from build123d import *

# Parameters (mm, degrees)
ESQUISSE1_R        = 1.5
ESQUISSE1_W        = 7.5
ESQUISSE1_H        = 5
BOSS_EXTRU_1_DEPTH = 5


with BuildPart() as part:
    # Esquisse1 → Boss.-Extru.1 (new body)
    with BuildSketch(Plane.XY):
        with BuildLine():
            Line((40, -6), (0, -6))
            ThreePointArc((0, -6), (-6, 0), (0, 6))
            Line((0, 6), (40, 6))
            ThreePointArc((40, 6), (46, 0), (40, -6))
        make_face()
        with Locations((40, 0)):
            Circle(ESQUISSE1_R, mode=Mode.SUBTRACT)
        Circle(ESQUISSE1_R, mode=Mode.SUBTRACT)
        with Locations((26.25, 0)):
            Rectangle(ESQUISSE1_W, ESQUISSE1_H, mode=Mode.SUBTRACT)
        with Locations((13.75, 0)):
            Rectangle(ESQUISSE1_W, ESQUISSE1_H, mode=Mode.SUBTRACT)
    extrude(amount=BOSS_EXTRU_1_DEPTH)


solid = part.part
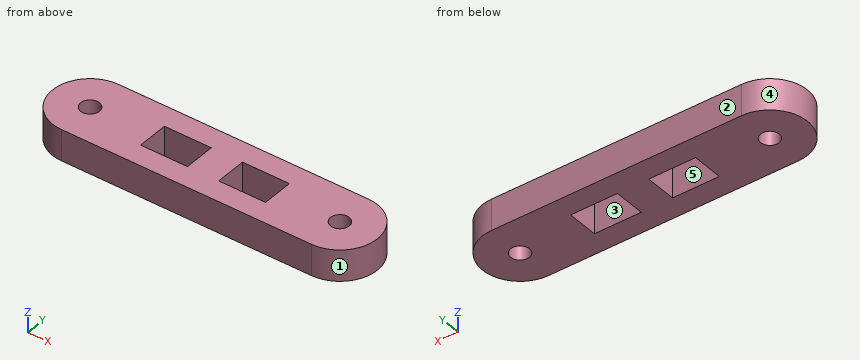
For this review, take the finished solid that the model builds, in its own axes (mm). Face numbers are marked on the shaded views. A direction names the side the tool comes from. Give positions to 0.01 mm unless a question says otherwise; leave off trailing zeros. Loops run counter-clockwise (first coordinate to the right, second up) from the corner with the lowest first, then second, coordinate; pieces in that order, holes last. Notation, with made-up numbers: M -25,45.25 L 10,45.25 A16 ccw 10,59.25 Z; hole C 76,49.5 d1. An arc over 180 degrees is marked long. Answer as a JSON object with one key per item and string values. Group by question number.
Q1. Add section A-A on y = 0. Give the boundary of the cut face in (x, z), and give its area (3 significant figures).
Q2. Tool access review of the marked faces 4 and 5: name each direction out of +Z, -Z, +X, -X, +Y, -Y from which nothing blocks a thin tool from reaching the whole face with its end or side.
Q3. Add section C-C on z = 3.45. Give the boundary of the cut face in (x, y), and give its area (3 significant figures).
Q4. Add section B-B on x = 29. Give the boundary of the cut face in (y, z).
Q5. For probe 1 along Y at (x, z) = (12.5, 3.85); probe 2 along Y at (x, z) = (40, 2.7); probe 3 along X at (y, z) = (0.5, 3.7), list the stretches that pass through material, from the lowest coordinate up. Write a range as [from, to].
Q6. Mouldability with a two-part tool opening along X and no side actions: class the marked faces 1, 2 and 3 as +X half, -X half, draft (parallel to the pull), parting line (faces both ways), or undercut.
Q7. Add section D-D on x = 39.5. Give the boundary of the cut face in (y, z).
Q8. Insertion check: P1, Ø1.5, axis at y = 1.5, z = 1, coming from the +X side; P2, Ø1, axis at y = 4.5, z = 4, coming from the +X side; P3, Ø2.5, axis at x = 0, y = 0, coming from the +Z side. Each pin has a flat end and moves straight along its axis. Give the tip position at first contact, or say it passes through.
Checked values:
{
 "1": {"outline": "M -6,0 L -1.5,0 L -1.5,5 L -6,5 Z; M 1.5,0 L 10,0 L 10,5 L 1.5,5 Z; M 17.5,0 L 22.5,0 L 22.5,5 L 17.5,5 Z; M 30,0 L 38.5,0 L 38.5,5 L 30,5 Z; M 41.5,0 L 46,0 L 46,5 L 41.5,5 Z", "area": "155 mm²"},
 "2": {"face 4": "+Z, -Z, -X", "face 5": "+Z, -Z"},
 "3": {"outline": "M 0,-6 L 40,-6 A6 ccw 40,6 L 0,6 A6 ccw Z; hole C 0,0 d3; hole M 10,-2.5 L 17.5,-2.5 L 17.5,2.5 L 10,2.5 Z; hole M 22.5,-2.5 L 30,-2.5 L 30,2.5 L 22.5,2.5 Z; hole C 40,0 d3", "area": "504 mm²"},
 "4": {"outline": "M -6,0 L -2.5,0 L -2.5,5 L -6,5 Z; M 2.5,0 L 6,0 L 6,5 L 2.5,5 Z"},
 "5": {"probe 1": "[-6, -2.5], [2.5, 6]", "probe 2": "[-6, -1.5], [1.5, 6]", "probe 3": "[-5.98, -1.41], [1.41, 10], [17.5, 22.5], [30, 38.59], [41.41, 45.98]"},
 "6": {"face 1": "+X half", "face 2": "draft", "face 3": "undercut"},
 "7": {"outline": "M -6,0 L -1.41,0 L -1.41,5 L -6,5 Z; M 1.41,0 L 6,0 L 6,5 L 1.41,5 Z"},
 "8": {"P1": "x = 45.95", "P2": "x = 44.47", "P3": "through"}
}
